Print and shaded views of the part. All mm, measured from the part's lowest x, y and z. Coordinates: 2 decimals unless noted, no trailing zeros. Order: outer loops, then holes, each group sorted by start corner. A loop starts at its lowest first (then second) coordinate and runs counter-clockwise, first axis right, second up. Notation, with made-up numbers: (81.25, 41.25) - (138.25, 41.25) arc R29 ccw to (138.25, 72.25) - close; hole circle Ø8 at (71, -34.75). An arc over 180 degrees is marked (long way). Write each question's results on one line, items separated by ' | '.
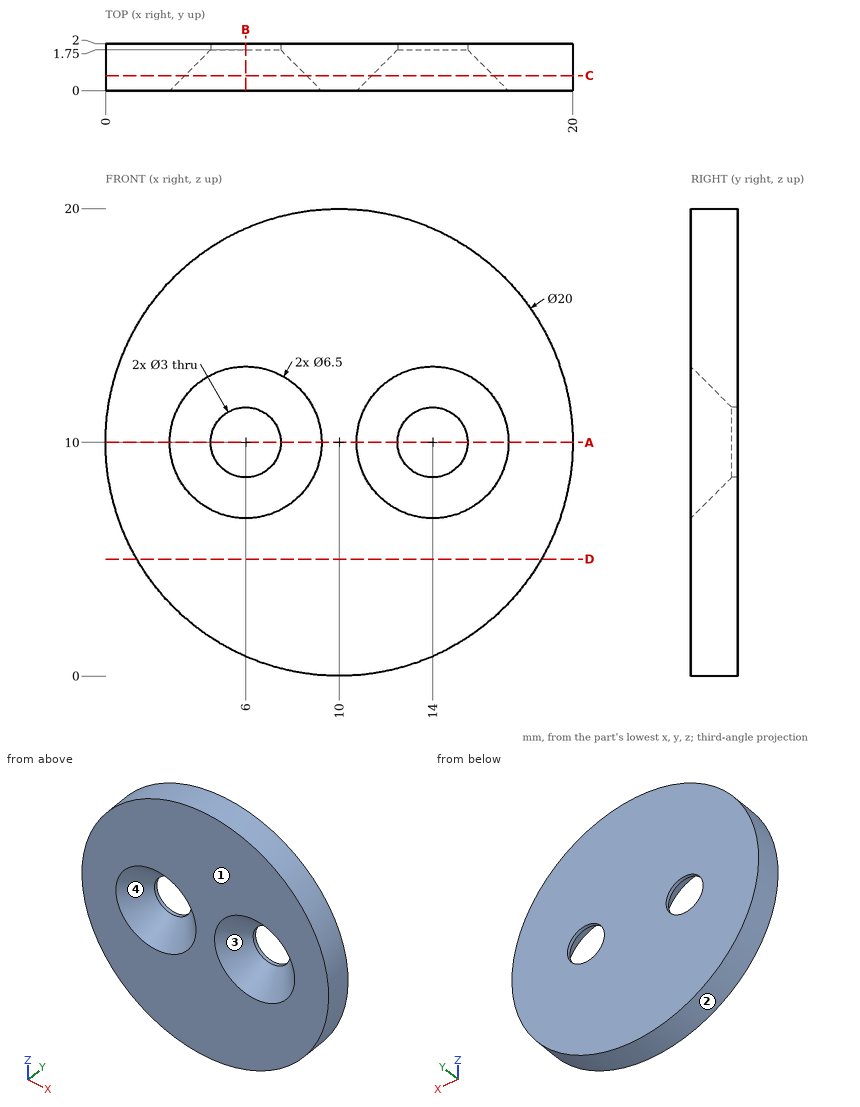
1. Drop flat-ended pins along their axis: pin 1 Ø4 at (x, z) = (6, 10) entering from -Y; pin 2 Ø1.8 at (x, z) = (14, 10) entering from +Y. Give the stop position or say it passes through.
Solved:
pin 1: stops at y = 1.25 | pin 2: passes through
2. Band-saw the part on A-A on z = 10. Give the cut face in (x, y), then the cut area to 3 significant figures.
Solved:
outline: (0, 0) - (2.75, 0) - (4.5, 1.75) - (4.5, 2) - (0, 2) - close; (7.5, 1.75) - (9.25, 0) - (10.75, 0) - (12.5, 1.75) - (12.5, 2) - (7.5, 2) - close; (15.5, 1.75) - (17.25, 0) - (20, 0) - (20, 2) - (15.5, 2) - close | area: 21.9 mm2
3. Two-plate mould, pull along X, no slides. Class the marked faces 1, 2, 3 and 4: +X half, -X half, draft (parallel to the pull), parting line (faces both ways), or undercut.
Solved:
face 1: draft | face 2: parting line | face 3: undercut | face 4: undercut
4. Band-saw the part on C-C on y = 0.65. Give the cut face in (x, z), then the cut area to 3 significant figures.
Solved:
outline: circle Ø20 at (10, 10); hole circle Ø5.2 at (6, 10); hole circle Ø5.2 at (14, 10) | area: 272 mm2
5. Probe line 1 (X direction, y = 1.9, z = 10); line 2 (X direction, y = 0.7, z = 10.25); line 3 (Z direction, x = 12.75, y = 0.55). List the from-to ranges inside material, lowest first.
Solved:
line 1: x = 0 to 4.5, 7.5 to 12.5, 15.5 to 20 | line 2: x = 0 to 3.46, 8.54 to 11.46, 16.54 to 20 | line 3: z = 0.39 to 7.61, 12.39 to 19.61
6. Band-saw the part on D-D on z = 5. Give the cut face in (x, y).
Solved:
outline: (1.34, 0) - (18.66, 0) - (18.66, 2) - (1.34, 2) - close
7. Band-saw the part on B-B on x = 6. Give the cut face in (y, z), then the cut area to 3 significant figures.
Solved:
outline: (0, 0.83) - (2, 0.83) - (2, 8.5) - (1.75, 8.5) - (0, 6.75) - close; (0, 13.25) - (1.75, 11.5) - (2, 11.5) - (2, 19.17) - (0, 19.17) - close | area: 27.6 mm2
